Verification items for the finished model (mm, model axes). A direction names the side the tool comes from. Give positions to 0.01 mm unless a question says otherwise; leave off trailing zeros. Order: outer loops, then holes, each group sorted by start corner. A loop starts at its lowest first (then second) coordinate and runs counter-clockwise, first axis right, second up.
from build123d import *

# Parameters (mm, degrees)
BOSS_EXTRUDE1_DEPTH = 107.95
CUT_EXTRUDE1_REACH  = 115.103
SKETCH2_R           = 3.175


with BuildPart() as part:
    # Sketch1 → Boss-Extrude1 (new body)
    with BuildSketch(Plane.XY):
        Polygon((0, 0), (25.4, 0), (25.4, -25.4), (22.225, -25.4), (22.225, -3.175), (0, -3.175), align=None)
    extrude(amount=BOSS_EXTRUDE1_DEPTH)

    # Sketch2 → Cut-Extrude1 (cut, up to next)
    with BuildSketch(Plane.XZ.offset(3.175), mode=Mode.PRIVATE) as cut_extrude1_sk1:
        with Locations(Location((12.7, 12.7, 0), (0, 0, 270))):
            Circle(SKETCH2_R)
    cut_extrude1_tool1 = extrude(cut_extrude1_sk1.sketch, amount=-CUT_EXTRUDE1_REACH, mode=Mode.PRIVATE) & part.part
    # Sketch2 → Cut-Extrude1 (cut, up to next)
    with BuildSketch(Plane.XZ.offset(3.175), mode=Mode.PRIVATE) as cut_extrude1_sk2:
        with Locations(Location((12.7, 95.25, 0), (0, 0, 270))):
            Circle(SKETCH2_R)
    cut_extrude1_tool2 = extrude(cut_extrude1_sk2.sketch, amount=-CUT_EXTRUDE1_REACH, mode=Mode.PRIVATE) & part.part
    add(cut_extrude1_tool1.solids().sort_by_distance((12.7, -3.175, 12.7))[0], mode=Mode.SUBTRACT)
    add(cut_extrude1_tool2.solids().sort_by_distance((12.7, -3.175, 95.25))[0], mode=Mode.SUBTRACT)


solid = part.part
(1) Section check C-C, the plane z = 67.5. Enter the section's corners in (x, y) (3 decimals).
Solved:
outline: (0, -3.175) - (22.225, -3.175) - (22.225, -25.4) - (25.4, -25.4) - (25.4, 0) - (0, 0) - close
(2) Scan lines: line 1 (X direction, y = -1.85, z = 12.7) (3 decimals); line 2 (X direction, y = -15.75, z = 18) (3 decimals); line 3 (Y direction, x = 14.5, z = 38) (3 decimals). Record each from-to range of solid material in increasing order.
Solved:
line 1: x = 0 to 9.525, 15.875 to 25.4
line 2: x = 22.225 to 25.4
line 3: y = -3.175 to 0
(3) Release check for a two-part mould opening along Z. For faces 1 (the cylindrical face through (13.65, -1.61, 92.22)), 2 (the flat face through (23, -7, 107.95)), 3 (the flat face through (23, -7, 0)), 4 (the flat face through (0, -2, 53)) record: pulls with the +Z half, pulls with the -Z half, needs draft (parallel to the pull), parting line crosses it, or undercut.
Solved:
face 1: undercut
face 2: pulls with the +Z half
face 3: pulls with the -Z half
face 4: needs draft
(4) Section check B-B, the plane x = 12.7. Enter the section's corners in (y, z) (3 decimals).
Solved:
outline: (-3.175, 0) - (0, 0) - (0, 9.525) - (-3.175, 9.525) - close; (-3.175, 15.875) - (0, 15.875) - (0, 92.075) - (-3.175, 92.075) - close; (-3.175, 98.425) - (0, 98.425) - (0, 107.95) - (-3.175, 107.95) - close
(5) Go/stop test with flat-tipped pins: pin 1 (1.5 mm diameter, centred on y = -16.5, z = 82.5, fed in from -X) (3 decimals); pin 2 (5 mm diameter, centred on x = 12.7, z = 12.7, fed in from +Y). Record where each tip stops, or that it passes through.
Solved:
pin 1: stops at x = 22.225
pin 2: passes through
(6) Section check D-D, the plane x = 2.5. Enter the section's corners in (y, z) (3 decimals).
Solved:
outline: (-3.175, 0) - (0, 0) - (0, 107.95) - (-3.175, 107.95) - close
(7) Set-up check for faces 5 (the flat face through (24, -25.4, 53)), 6 (the flat face through (22.225, -14, 53)): record each of +Z, -Z, +X, -X, +Y, -Y from which the full face is reachable in a straight line by a thin tool's end or side.
Solved:
face 5: +Z, -Z, +X, -X, -Y
face 6: +Z, -Z, -X, -Y
(8) Section check A-A, the plane z = 95.25. Enter the section's corners in (x, y) (3 decimals), then the cut area to 3 significant figures.
Solved:
outline: (0, -3.175) - (9.525, -3.175) - (9.525, 0) - (0, 0) - close; (15.875, -3.175) - (22.225, -3.175) - (22.225, -25.4) - (25.4, -25.4) - (25.4, 0) - (15.875, 0) - close
area: 131 mm2
